Source: three-view drawing plus pictorial views. Frame: mm from the lowest corner of the part. Round coordinates to 2 decimals unless told otherwise and drop trailing zeros. Write each loop counter-clockwise with the first axis right and the second up, starting at its lowest first coordinate (ties: lowest second). Pieces come first, ordered by that corner, then holes.
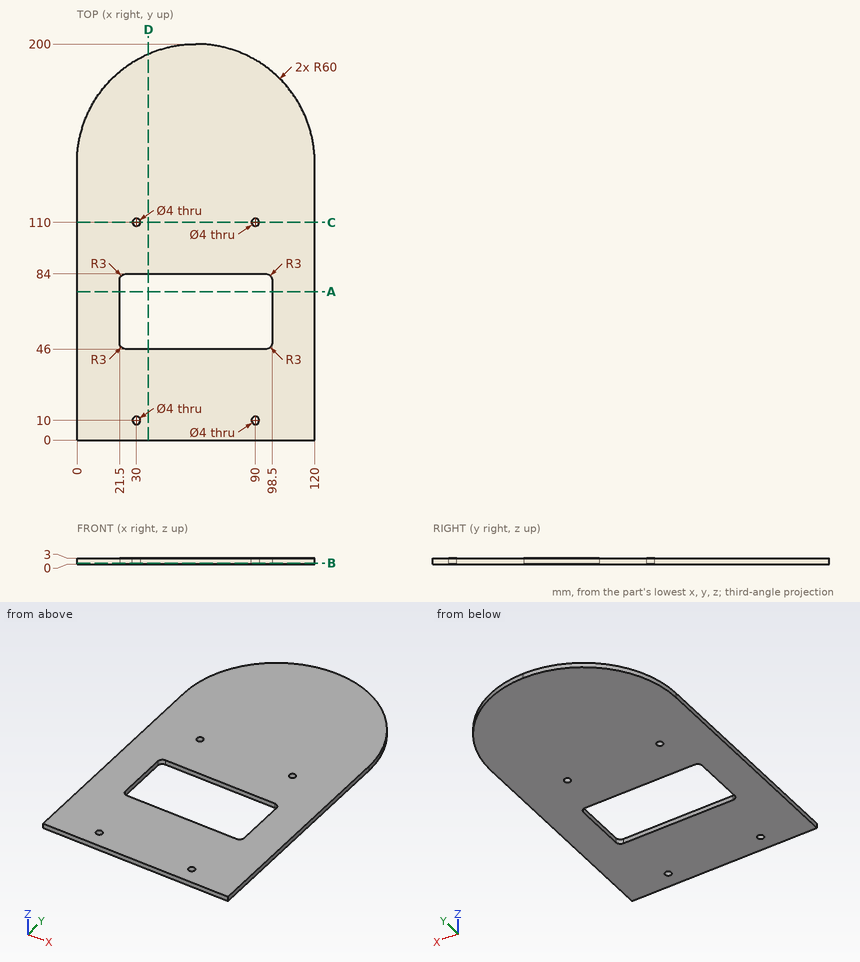
1) First-contact query: P1, Ø1, axis at x = 101.5, z = 1.5, coming from the +Y side; P2, Ø1.5, axis at x = 74, z = 2, coming from the +Y side; P3, Ø6.5, axis at x = 90, y = 110, coming from the +Z side. Flat tips, straight axial feed; report the tip coordinate or a pass-through.
2) Section A-A on y = 75. Output: boundary loops of the cut face in (x, z).
3) Line query: probe 1 along X at (y, z) = (57, 1.6); probe 2 along Y at (x, z) = (90, 0.85); probe 3 along Y at (x, z) = (82, 0.8). Output: solid intervals per line, ascending.
4) Section D-D on x = 36. Output: boundary loops of the cut face in (y, z).
5) Section C-C on y = 110. Output: boundary loops of the cut face in (x, z), plus the area to 3 significant figures.
6) Section B-B on z = 0.6. State how many separate pieces and enclosed holes the cut face has, plus the area to 3 significant figures.
Filled in:
1. P1: stops at y = 183.81
1. P2: stops at y = 198.52
1. P3: stops at z = 3
2. outline: (0, 0) - (21.5, 0) - (21.5, 3) - (0, 3) - close; (98.5, 0) - (120, 0) - (120, 3) - (98.5, 3) - close
3. probe 1: x = 0 to 21.5, 98.5 to 120
3. probe 2: y = 0 to 8, 12 to 46, 84 to 108, 112 to 191.96
3. probe 3: y = 0 to 46, 84 to 195.82
4. outline: (0, 0) - (46, 0) - (46, 3) - (0, 3) - close; (84, 0) - (194.99, 0) - (194.99, 3) - (84, 3) - close
5. outline: (0, 0) - (28, 0) - (28, 3) - (0, 3) - close; (32, 0) - (88, 0) - (88, 3) - (32, 3) - close; (92, 0) - (120, 0) - (120, 3) - (92, 3) - close
5. area: 336 mm2
6. separate pieces: 1
6. enclosed holes: 5
6. area: 19,500 mm2
